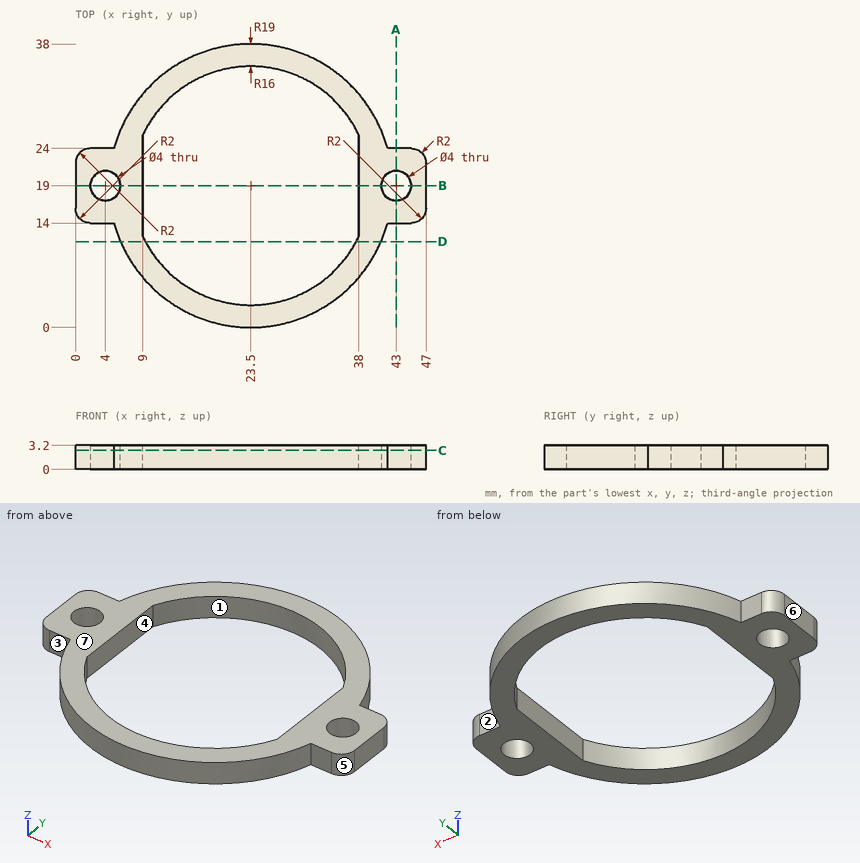
Input: dimensioned drawing with shaded views. Units: mm. Origin: part minimum x, y, z. A direction names the side the tool comes from. Round coordinates to 2 decimals unless told otherwise and drop trailing zeros. Order: outer loops, then holes, each group sorted by start corner. A loop starts at its lowest first (then second) coordinate and runs counter-clockwise, first axis right, second up.
Q1. Pin query (flat end, axial travel): pin 1 (3 mm diameter, centred on x = 4, y = 19, fed in from -Z); pin 2 (1 mm diameter, centred on x = 43.5, z = 1.5, fed in from +Y). Return the tip coordinate at first contact, or that it passes through.
Result sheet:
pin 1: passes through
pin 2: stops at y = 24
Q2. Section A-A, the plane x = 43. Output: boundary loops of the cut face in (y, z).
Result sheet:
outline: (14, 0) - (17, 0) - (17, 3.2) - (14, 3.2) - close; (21, 0) - (24, 0) - (24, 3.2) - (21, 3.2) - close
Q3. Section C-C, the plane z = 2.55. Output: boundary loops of the cut face in (x, y).
Result sheet:
outline: (0, 16) arc R2 ccw to (2, 14) - (5.17, 14) arc R19 ccw to (41.83, 14) - (45, 14) arc R2 ccw to (47, 16) - (47, 22) arc R2 ccw to (45, 24) - (41.83, 24) arc R19 ccw to (5.17, 24) - (2, 24) arc R2 ccw to (0, 22) - close; hole circle Ø4 at (4, 19); hole (9, 12.24) arc R16 ccw to (38, 12.24) - (38, 25.76) arc R16 ccw to (9, 25.76) - close; hole circle Ø4 at (43, 19)
Q4. Mould query, pull axis X, two halves, no side actions, for the marked faces 4, 5, 6 and 7. Classes: released by +X, released by -X, zero draft, split by the parting line, or undercut.
Result sheet:
face 4: undercut
face 5: released by +X
face 6: released by -X
face 7: zero draft
Q5. Section B-B, the plane y = 19. Output: boundary loops of the cut face in (x, z).
Result sheet:
outline: (0, 0) - (2, 0) - (2, 3.2) - (0, 3.2) - close; (6, 0) - (9, 0) - (9, 3.2) - (6, 3.2) - close; (38, 0) - (41, 0) - (41, 3.2) - (38, 3.2) - close; (45, 0) - (47, 0) - (47, 3.2) - (45, 3.2) - close
Q6. Material intervals for probe 1 along X at (y, z) = (19, 1.1); probe 2 along Y at (x, z) = (4, 1.35); probe 3 along Y at (x, z) = (23, 0.3), sorted ascending.
Result sheet:
probe 1: x = 0 to 2, 6 to 9, 38 to 41, 45 to 47
probe 2: y = 14 to 17, 21 to 24
probe 3: y = 0.01 to 3.01, 34.99 to 37.99
Q7. Access query for the marked faces 1, 2 and 3. Directions: +Z, -Z, +X, -X, +Y, -Y. A direction counts if a zero-diameter tool reaches every point of the face in a straight line with its end or side. Return the directions, or none.
Result sheet:
face 1: +Z, -Z
face 2: +Z, -Z, +X, +Y
face 3: +Z, -Z, -X, -Y
Q8. Section D-D, the plane y = 11.5. Output: boundary loops of the cut face in (x, z).
Result sheet:
outline: (6.04, 0) - (9.37, 0) - (9.37, 3.2) - (6.04, 3.2) - close; (37.63, 0) - (40.96, 0) - (40.96, 3.2) - (37.63, 3.2) - close
